Here's how the part is built. I have some questions about the finished solid (model axes, mm). Round coordinates to 2 decimals unless told otherwise and drop trailing zeros. Loops run counter-clockwise (first coordinate to the right, second up) from the corner with the lowest first, then second, coordinate; pieces in that order, holes last. Notation, with made-up numbers: M 23.25,-21 L 28.25,-21 A19 ccw 28.25,7 Z; hole C -0.5,-4 d2. An arc over 180 degrees is marked long. Write each question's results on one line, items separated by ' | '. Start each with the question number.
```python
from build123d import *

# Parameters (mm, degrees)
SKETCH1_W           = 6.35
SKETCH1_H           = 12.446
SKETCH1_W_2         = 12.446
SKETCH1_H_2         = 6.35
SKETCH1_H_3         = 12.573
BOSS_EXTRUDE1_DEPTH = 6.35


with BuildPart() as part:
    # Sketch1 → Boss-Extrude1 (new body)
    with BuildSketch(Plane(origin=(0, 0, 0), x_dir=(1, 0, 0), z_dir=(0, 1, 0))):
        with BuildLine():
            Line((19.177, -311.15), (247.777, -311.15))
            ThreePointArc((247.777, -311.15), (283.698024484, -296.271024484), (298.577, -260.35))
            Line((298.577, -260.35), (298.577, -31.75))
            ThreePointArc((298.577, -31.75), (283.698024484, 4.171024484), (247.777, 19.05))
            Line((247.777, 19.05), (19.177, 19.05))
            ThreePointArc((19.177, 19.05), (-16.744024484, 4.171024484), (-31.623, -31.75))
            Line((-31.623, -31.75), (-31.623, -260.35))
            ThreePointArc((-31.623, -260.35), (-16.744024484, -296.271024484), (19.177, -311.15))
        make_face()
        with Locations((-9.398, -234.95)):
            Rectangle(SKETCH1_W, SKETCH1_H, mode=Mode.SUBTRACT)
        with Locations((-9.398, -209.55)):
            Rectangle(SKETCH1_W, SKETCH1_H, mode=Mode.SUBTRACT)
        with Locations((-9.398, -184.15)):
            Rectangle(SKETCH1_W, SKETCH1_H, mode=Mode.SUBTRACT)
        with Locations((-9.398, -158.75)):
            Rectangle(SKETCH1_W, SKETCH1_H, mode=Mode.SUBTRACT)
        with Locations((-9.398, -133.35)):
            Rectangle(SKETCH1_W, SKETCH1_H, mode=Mode.SUBTRACT)
        with Locations((-9.398, -107.95)):
            Rectangle(SKETCH1_W, SKETCH1_H, mode=Mode.SUBTRACT)
        with Locations((-9.398, -82.55)):
            Rectangle(SKETCH1_W, SKETCH1_H, mode=Mode.SUBTRACT)
        with Locations((-9.398, -57.15)):
            Rectangle(SKETCH1_W, SKETCH1_H, mode=Mode.SUBTRACT)
        with Locations((-9.398, -31.75)):
            Rectangle(SKETCH1_W, SKETCH1_H, mode=Mode.SUBTRACT)
        Polygon((-6.223, -12.573), (-12.573, -12.573), (-12.573, 0), (0, 0), (0, -6.35), (-6.223, -6.35), align=None, mode=Mode.SUBTRACT)
        Polygon((273.177, -285.75), (273.177, -279.527), (279.527, -279.527), (279.527, -292.1), (266.954, -292.1), (266.954, -285.75), align=None, mode=Mode.SUBTRACT)
        with Locations((276.352, -260.35)):
            Rectangle(SKETCH1_W, SKETCH1_H, mode=Mode.SUBTRACT)
        with Locations((276.352, -234.95)):
            Rectangle(SKETCH1_W, SKETCH1_H, mode=Mode.SUBTRACT)
        Polygon((-6.223, -279.527), (-6.223, -285.75), (0, -285.75), (0, -292.1), (-12.573, -292.1), (-12.573, -279.527), align=None, mode=Mode.SUBTRACT)
        with Locations((-9.398, -260.35)):
            Rectangle(SKETCH1_W, SKETCH1_H, mode=Mode.SUBTRACT)
        with Locations((276.352, -209.55)):
            Rectangle(SKETCH1_W, SKETCH1_H, mode=Mode.SUBTRACT)
        with Locations((276.352, -184.15)):
            Rectangle(SKETCH1_W, SKETCH1_H, mode=Mode.SUBTRACT)
        with Locations((276.352, -158.75)):
            Rectangle(SKETCH1_W, SKETCH1_H, mode=Mode.SUBTRACT)
        with Locations((276.352, -133.35)):
            Rectangle(SKETCH1_W, SKETCH1_H, mode=Mode.SUBTRACT)
        with Locations((276.352, -107.95)):
            Rectangle(SKETCH1_W, SKETCH1_H, mode=Mode.SUBTRACT)
        with Locations((276.352, -82.55)):
            Rectangle(SKETCH1_W, SKETCH1_H, mode=Mode.SUBTRACT)
        with Locations((276.352, -57.15)):
            Rectangle(SKETCH1_W, SKETCH1_H, mode=Mode.SUBTRACT)
        with Locations((276.352, -31.75)):
            Rectangle(SKETCH1_W, SKETCH1_H, mode=Mode.SUBTRACT)
        Polygon((279.527, -12.573), (273.177, -12.573), (273.177, -6.35), (266.954, -6.35), (266.954, 0), (279.527, 0), align=None, mode=Mode.SUBTRACT)
        with Locations((19.177, -3.175)):
            Rectangle(SKETCH1_W_2, SKETCH1_H_2, mode=Mode.SUBTRACT)
        with Locations((44.577, -3.175)):
            Rectangle(SKETCH1_W_2, SKETCH1_H_2, mode=Mode.SUBTRACT)
        with Locations((69.977, -3.175)):
            Rectangle(SKETCH1_W_2, SKETCH1_H_2, mode=Mode.SUBTRACT)
        with Locations((95.377, -3.175)):
            Rectangle(SKETCH1_W_2, SKETCH1_H_2, mode=Mode.SUBTRACT)
        with Locations((120.777, -3.175)):
            Rectangle(SKETCH1_W_2, SKETCH1_H_2, mode=Mode.SUBTRACT)
        with Locations((146.177, -3.175)):
            Rectangle(SKETCH1_W_2, SKETCH1_H_2, mode=Mode.SUBTRACT)
        with Locations((171.577, -3.175)):
            Rectangle(SKETCH1_W_2, SKETCH1_H_2, mode=Mode.SUBTRACT)
        with Locations((196.977, -3.175)):
            Rectangle(SKETCH1_W_2, SKETCH1_H_2, mode=Mode.SUBTRACT)
        with Locations((222.377, -3.175)):
            Rectangle(SKETCH1_W_2, SKETCH1_H_2, mode=Mode.SUBTRACT)
        with Locations((247.777, -3.175)):
            Rectangle(SKETCH1_W_2, SKETCH1_H_2, mode=Mode.SUBTRACT)
        with Locations((257.175, -158.5595)):
            Rectangle(SKETCH1_W, SKETCH1_H_3, mode=Mode.SUBTRACT)
        with Locations((257.175, -272.8595)):
            Rectangle(SKETCH1_W, SKETCH1_H_3, mode=Mode.SUBTRACT)
        with Locations((257.175, -44.2595)):
            Rectangle(SKETCH1_W, SKETCH1_H_3, mode=Mode.SUBTRACT)
        with Locations((9.779, -44.2595)):
            Rectangle(SKETCH1_W, SKETCH1_H_3, mode=Mode.SUBTRACT)
        with Locations((9.779, -158.5595)):
            Rectangle(SKETCH1_W, SKETCH1_H_3, mode=Mode.SUBTRACT)
        with Locations((9.779, -272.8595)):
            Rectangle(SKETCH1_W, SKETCH1_H_3, mode=Mode.SUBTRACT)
    extrude(amount=BOSS_EXTRUDE1_DEPTH)


solid = part.part
```
Item 1: If we section it at A-A on x = 120: Please give me the cut outline in (y, z), and give its area (3 significant figures).
Item 2: I need wall thicknesses on L1, parallel to X at y = 3, z = 178.5; L2, parallel to X at y = 1, z = 12.5; L3, parallel to Z at x = 97.5, y = 3.25. Which ranges of each line are inside material? Lowest first, please.
Item 3: I'm going to push flat-ended pins straight in: pin 1 (1.9 mm diameter, centred on x = 278, y = 2.5, fed in from +Z); pin 2 (1.9 mm diameter, centred on y = 4.5, z = 271, fed in from -X). Where does each tip first touch, or does it pass through?
Item 4: If we section it at B-B on z = 133: Please give me the cut outline in (x, y), and give its area (3 significant figures).
Item 5: If we section it at C-C on y = 3.5: Count the separate pieces of the cut face and the enclosed holes in it, and give its area (3 significant figures).
Numbers:
1) outline: M 0,-19.05 L 6.35,-19.05 L 6.35,0 L 0,0 Z; M 0,6.35 L 6.35,6.35 L 6.35,311.15 L 0,311.15 Z | area: 2,060 mm²
2) L1: -31.62 to -12.57, -6.22 to 273.18, 279.53 to 298.58 | L2: -27.83 to -12.57, -6.22 to 273.18, 279.53 to 294.79 | L3: -19.05 to 0, 6.35 to 311.15
3) pin 1: z = 301.87 | pin 2: x = -30.69
4) outline: M -31.62,0 L -12.57,0 L -12.57,6.35 L -31.62,6.35 Z; M -6.22,0 L 273.18,0 L 273.18,6.35 L -6.22,6.35 Z; M 279.53,0 L 298.58,0 L 298.58,6.35 L 279.53,6.35 Z | area: 2,020 mm²
5) separate pieces: 1 | enclosed holes: 40 | area: 103,000 mm²
